Geometry check sheet. Reference: the model listing, model coordinates, mm. Face numbers are marked on the shaded views. Coordinates: 2 decimals unless noted, no trailing zeros. Loops run counter-clockwise (first coordinate to the right, second up) from the corner with the lowest first, then second, coordinate; pieces in that order, holes last.
from build123d import *

# Parameters (mm, degrees)
SKETCH_1_W      = 80
SKETCH_1_H      = 300
EXTRUDE_1_DEPTH = 10
SKETCH_2_W      = 80
SKETCH_2_H      = 10
EXTRUDE_2_DEPTH = 20
CHAMFER_1_SIZE  = 2.5


with BuildPart() as part:
    # 草圖1 → 填料-伸長1 (new body)
    with BuildSketch(Plane.XY):
        with Locations((78.435797513, 9.285783834)):
            Rectangle(SKETCH_1_W, SKETCH_1_H)
    extrude(amount=-EXTRUDE_1_DEPTH)

    # 草圖2 → 填料-伸長2 (add)
    with BuildSketch(Plane.XY):
        with Locations((78.435797513, -135.714216166)):
            Rectangle(SKETCH_2_W, SKETCH_2_H)
        with Locations((78.435797513, 154.285783834)):
            Rectangle(SKETCH_2_W, SKETCH_2_H)
    extrude(amount=EXTRUDE_2_DEPTH)

    # 導角1
    chamfer_1_edges = [part.edges().sort_by_distance(p)[0] for p in [
        (118.435797513, 9.285783834, -10),
        (78.435797513, 159.285783834, -10),
        (78.435797513, -140.714216166, 20),
        (78.435797513, 159.285783834, 20),
        (38.435797513, 9.285783834, -10),
        (78.435797513, -140.714216166, -10),
        (38.435797513, 159.285783834, 5),
        (118.435797513, 159.285783834, 5),
        (118.435797513, -140.714216166, 5),
        (38.435797513, -140.714216166, 5),
    ]]
    chamfer(chamfer_1_edges, length=CHAMFER_1_SIZE)


solid = part.part
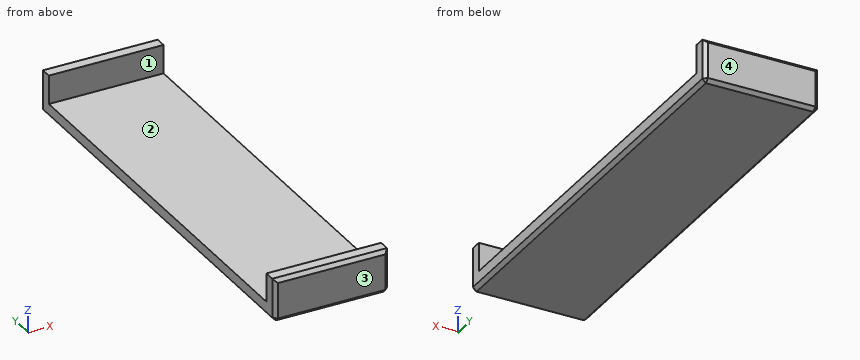
1) Material ranges on probe 1 along Y at (x, z) = (70, 8.5); probe 2 along Z at (x, y) = (115, -7); probe 3 along Y at (x, z) = (108, 19), recorded low to high.
Data:
probe 1: y = -140.71 to -130.71, 149.29 to 159.29
probe 2: z = -10 to 0
probe 3: y = -139.21 to -130.71, 149.29 to 157.79
2) Mould release check, pull along Y, two halves, no side actions. Record for the marked faces 1, 2, 3 and 4: +Y half, -Y half, draft (parallel to the pull), parting line (faces both ways), or undercut.
Data:
face 1: undercut
face 2: undercut
face 3: -Y half
face 4: +Y half
3) Section check A-A on z = 2.5. Record the cut outline in (x, y), and give its area (3 significant figures).
Data:
outline: (38.44, -138.21) - (40.94, -140.71) - (115.94, -140.71) - (118.44, -138.21) - (118.44, -130.71) - (38.44, -130.71) - close; (38.44, 149.29) - (118.44, 149.29) - (118.44, 156.79) - (115.94, 159.29) - (40.94, 159.29) - (38.44, 156.79) - close
area: 1,590 mm2
4) Section check B-B on x = 110.5. Record the cut outline in (y, z).
Data:
outline: (-140.71, -7.5) - (-138.21, -10) - (156.79, -10) - (159.29, -7.5) - (159.29, 17.5) - (156.79, 20) - (149.29, 20) - (149.29, 0) - (-130.71, 0) - (-130.71, 20) - (-138.21, 20) - (-140.71, 17.5) - close
5) Section check C-C on y = 64.5. Record the cut outline in (x, z).
Data:
outline: (38.44, -7.5) - (40.94, -10) - (115.94, -10) - (118.44, -7.5) - (118.44, 0) - (38.44, 0) - close
6) Depth check by flat-ended pin: pin 1 (5 mm diameter, centred on x = 96, y = 122, fed in from +Z). Enter the tip coordinate at first touch or a pass-through.
Data:
pin 1: stops at z = 0
